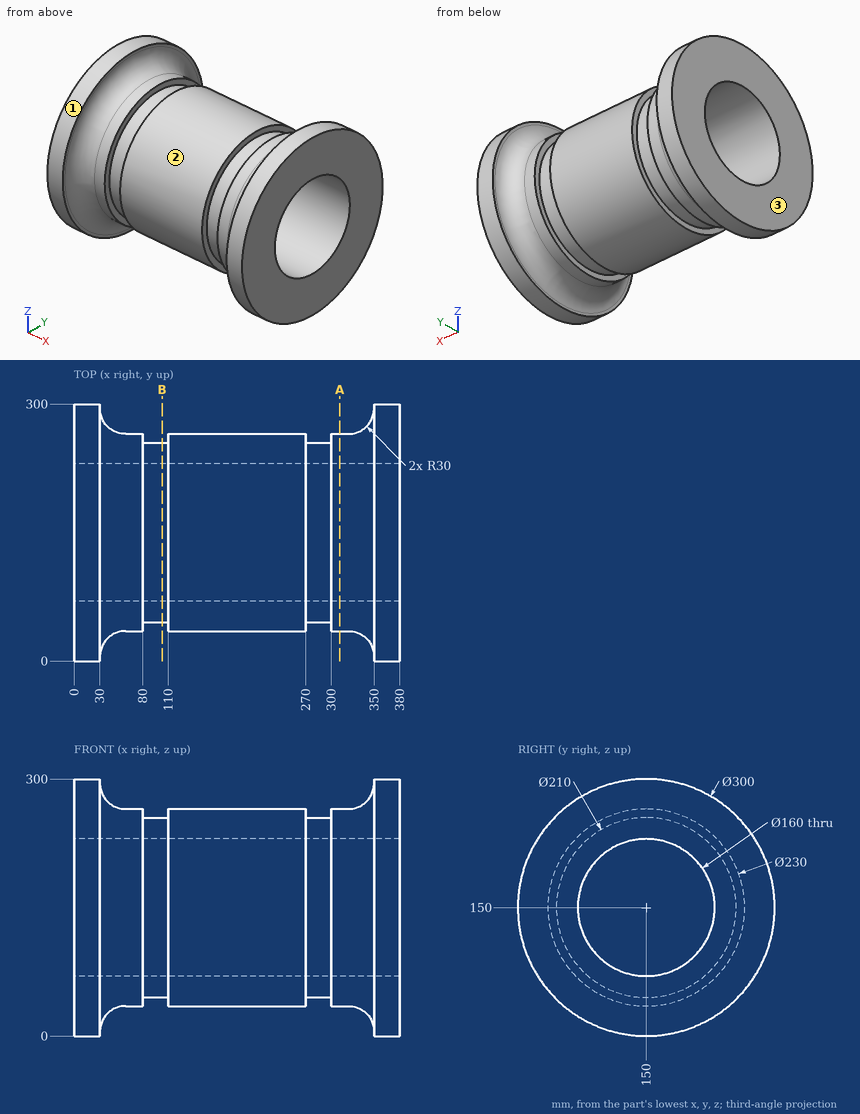
Job drawing, mm, ordinate dimensions from the low corner. One solid piece. Coordinates: 2 decimals unless noted, no trailing zeros. Write each loop counter-clockwise with the first axis right and the second up, starting at its lowest first coordinate (ties: lowest second). Pieces come first, ordered by that corner, then holes. Notation, with made-up numbers: (67.25, 66) - (124.25, 66) arc R15 cw to (124.25, 72) - close; hole circle Ø1 at (-12, 47.25). An arc over 180 degrees is marked (long way). Use a Markdown table: item, result. Add a question column.
Item 1: Band-saw the part on B-B, the plane x = 102.5. Give the cut face in (y, z).
Item 2: Mould opens along X. For the marked faces 1, 2 and 3 say: pulls with the +X half, pulls with the -X half, needs draft (parallel to the pull), parting line crosses it, or undercut.
Item 3: Band-saw the part on A-A, the plane x = 310. Give the cut face in (y, z), and give its area (3 significant figures).
Item 4: Flat gauge pins, fed straight in: pin 1 (6 mm diameter, centred on x = 190, y = 80.5, fed in from +Z); pin 2 (3 mm diameter, centred on x = 94, y = 129.5, fed in from -Z); pin 3 (1.5 mm diameter, centred on x = 220.5, z = 204.5, fed in from +Y). Where does each tip first touch, or does it go through?
Item 5: Drill centre lines: L1, parallel to X at y = 240.5, z = 205.5; L2, parallel to Y at x = 153, z = 150. Where is each one in solid material? Low to high. Write a range as from..to.
Numbers:
| question | item | result |
|---|---|---|
| 1 | outline | circle Ø210 at (150, 150); hole circle Ø160 at (150, 150) |
| 2 | face 1 | needs draft |
| 2 | face 2 | undercut |
| 2 | face 3 | pulls with the -X half |
| 3 | outline | circle Ø230 at (150, 150); hole circle Ø160 at (150, 150) |
| 3 | area | 21,400 mm2 |
| 4 | pin 1 | z = 243.82 |
| 4 | pin 2 | z = 46.73 |
| 4 | pin 3 | y = 251.67 |
| 5 | L1 | 0..80, 110..270, 300..380 |
| 5 | L2 | 35..70, 230..265 |
